Input: part model. Units: mm. Frame: model coordinates. Face numbers are marked on the shaded views. Give positions to 0.01 mm unless a question says otherwise; leave off trailing zeros. Order: outer loops, then holes, each group sorted by start corner. A loop starts at its lowest first (then second) coordinate and runs counter-clockwise, first axis right, second up. Notation, with made-up numbers: M 10,29 L 45,29 A29 ccw 45,51 Z; hole C 31,54 d1. An arc over 180 degrees is marked long. Use a Markdown table: item, result.
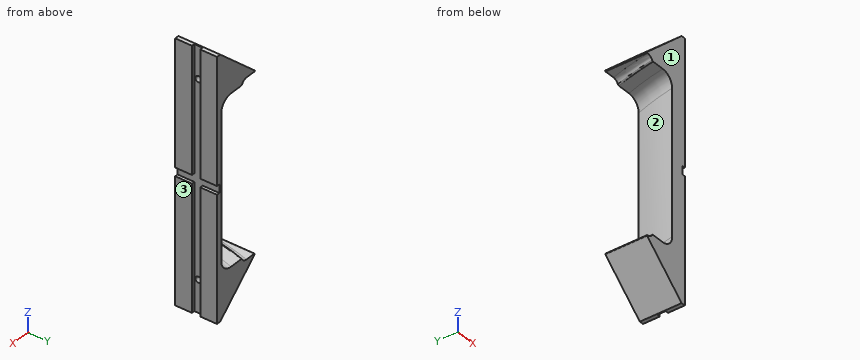
from build123d import *

# Parameters (mm, degrees)
F4_DEPTH  = 294.8
F6_DEPTH  = 70
F8_DEPTH  = 5
F9_R      = 5
F10_DEPTH = 30
F11_R     = 1


with BuildPart() as f2:
    # F2: sweep along a path in F1
    with BuildLine(Plane.XY) as f2_path:
        ThreePointArc((-415.6921938165, 240), (-463.6443966188, 124.2331416492), (-480, 0))
    # F0 (on Front) → F2 (sweep)
    with BuildSketch(Plane.XZ):
        with BuildLine():
            Line((-480, 120.4), (-480, 0))
            Line((-480, 0), (-480, -120.4))
            ThreePointArc((-480, -120.4), (-485.8578643763, -134.5421356237), (-500, -140.4))
            Line((-500, -140.4), (-520.7750278397, -140.4))
            ThreePointArc((-520.7750278397, -140.4), (-522.0979034952, -140.7786796564), (-523.0200222717, -141.8))
            ThreePointArc((-523.0200222717, -141.8), (-526.7084973779, -145.8852813742), (-532, -147.4))
            Line((-532, -147.4), (-450.85, -147.4))
            Line((-450.85, -147.4), (-450.85, 0))
            Line((-450.85, 0), (-450.85, 147.4))
            Line((-450.85, 147.4), (-532, 147.4))
            ThreePointArc((-532, 147.4), (-526.7084973779, 145.8852813742), (-523.0200222717, 141.8))
            ThreePointArc((-523.0200222717, 141.8), (-522.0979034952, 140.7786796564), (-520.7750278397, 140.4))
            Line((-520.7750278397, 140.4), (-500, 140.4))
            ThreePointArc((-500, 140.4), (-485.8578643763, 134.5421356237), (-480, 120.4))
        make_face()
    sweep(path=f2_path.line)

    # F3 (on face) → F4 (cut, through all)
    with BuildSketch(Plane.XY.offset(147.4)):
        with BuildLine():
            Line((-445, 85), (-525.1656881404, 85))
            ThreePointArc((-525.1656881404, 85), (-530.2886695427, 42.6371546266), (-532, 0))
            Line((-532, 0), (-450.85, 0))
            ThreePointArc((-450.85, 0), (-435.4876587824, 116.6885664845), (-390.4475532962, 225.425))
            Line((-390.4475532962, 225.425), (-460.7255148133, 266))
            ThreePointArc((-460.7255148133, 266), (-487.9888178112, 211.8747594482), (-508.9194435272, 155))
            Line((-508.9194435272, 155), (-445, 155))
            Line((-445, 155), (-445, 85))
        make_face()
    extrude(amount=-F4_DEPTH, mode=Mode.SUBTRACT)

    # F5 (on face) → F6 (join)
    with BuildSketch(Plane.XZ.offset(-85)):
        Polygon((-451.8080547159, 216.37), (-528.4069998637, 147.4), (-445, 147.4), (-445, 216.37), align=None)
        Polygon((-528.4069998637, -147.4), (-451.8080547159, -216.37), (-445, -216.37), (-445, -147.4), align=None)
    extrude(amount=-F6_DEPTH)

    # F7 (on face) → F8 (cut)
    with BuildSketch(Plane.YZ.offset(-445)):
        Polygon((127, 216.37), (113, 216.37), (113, 7), (85, 7), (85, -7), (113, -7), (113, -216.37), (127, -216.37), (127, -7), (155, -7), (155, 7), (127, 7), align=None)
    extrude(amount=-F8_DEPTH, mode=Mode.SUBTRACT)

    # F9 (on face) → F10 (cut)
    with BuildSketch(Plane.YZ.offset(-450)):
        with Locations((120, 162.5)):
            Circle(F9_R)
        with Locations((120, -162.5)):
            Circle(F9_R)
    extrude(amount=-F10_DEPTH, mode=Mode.SUBTRACT)

    # F11
    f11_edges = [f2.edges().sort_by_distance(p)[0] for p in [
        (-528.407, 120, 147.4),
        (-528.407, 120, -147.4),
    ]]
    fillet(f11_edges, radius=F11_R)


solid = f2.part
1) Cut plane C-C on z = -162.5. Return loops of the section in (x, y).
Response values:
| item | result |
|---|---|
| outline | M -511.64,85 L -445,85 L -445,113 L -450,113 L -450,115 L -480,115 L -480,125 L -450,125 L -450,127 L -445,127 L -445,155 L -511.64,155 Z |
2) Material intervals for line 1 (Y direction, x = -467, z = 162); line 2 (Z direction, x = -471.25, y = 120); line 3 (Z direction, x = -461.75, y = 120), sorted ascending. Write a range as from..to.
Response values:
| item | result |
|---|---|
| line 1 | y = 85..115.03, 124.97..155 |
| line 2 | z = -198.86..-167.5, -157.5..-134.96, 134.96..157.5, 167.5..198.86 |
| line 3 | z = -207.42..-167.5, -157.5..157.5, 167.5..207.42 |
3) Cut plane A-A on z = 28. Return loops of the section in (x, y), and give its area (3 significant figures).
Response values:
| item | result |
|---|---|
| outline | M -472.41,85 L -445,85 L -445,113 L -450,113 L -450,127 L -445,127 L -445,155 L -454.29,155 A480 ccw Z |
| area | 1,280 mm² |
4) First-contact query: pin 1 Ø13.5 at (x, y) = (-521, 103) entering from +Z; pin 2 Ø8 at (y, z) = (119, 161) entering from +X; pin 3 Ø1 at (y, z) = (129.5, -99) entering from -X; pin 4 Ø4 at (x, z) = (-509.5, -137.5) entering from -Y. Flat tips, straight axial feed; report the tip coordinate or a pass-through.
Response values:
| item | result |
|---|---|
| pin 1 | stops at z = 160.15 |
| pin 2 | stops at x = -450 |
| pin 3 | stops at x = -462.34 |
| pin 4 | passes through |
5) Cut plane B-B on x = -465. State how many separate pieces and enclosed holes the cut face has, and give its area (3 significant figures).
Response values:
| item | result |
|---|---|
| separate pieces | 1 |
| enclosed holes | 2 |
| area | 18,900 mm² |
6) Mould query, pull axis Y, two halves, no side actions, for the marked faces 1, 2 and 3. Classes: released by +Y, released by -Y, zero draft, split by the parting line, or undercut.
Response values:
| item | result |
|---|---|
| face 1 | released by -Y |
| face 2 | released by +Y |
| face 3 | zero draft |
